from build123d import *

# Parameters (mm, degrees)
SKETCH1_R           = 29.5
BOSS_EXTRUDE1_DEPTH = 1.75
SKETCH2_R           = 27.5
BOSS_EXTRUDE2_DEPTH = 4.45
SKETCH3_R           = 1.25
CUT_EXTRUDE1_DEPTH  = 43.470018837
CIRPATTERN1_COUNT   = 16


with BuildPart() as part:
    # Sketch1 → Boss-Extrude1 (new, symmetric)
    with BuildSketch(Plane(origin=(0, 0, 0), x_dir=(1, 0, 0), z_dir=(0, 1, 0))):
        with Locations(Location((0, 0, 0), (0, 0, 270))):
            Circle(SKETCH1_R)
    extrude(amount=BOSS_EXTRUDE1_DEPTH, both=True)

    # Sketch2 → Boss-Extrude2 (add)
    with BuildSketch(Plane(origin=(0, 1.75, 0), x_dir=(1, 0, 0), z_dir=(0, 1, 0))):
        with Locations(Location((0, 0, 0), (0, 0, 270))):
            Circle(SKETCH2_R)
    extrude(amount=BOSS_EXTRUDE2_DEPTH)

    # Sketch3 → Cut-Extrude1 (cut, through all)
    with BuildSketch(Plane.XZ.offset(1.75)):
        with Locations(Location((0, 23.75, 0), (0, 0, 270))):
            Circle(SKETCH3_R)
    cut_extrude1 = extrude(amount=-CUT_EXTRUDE1_DEPTH, mode=Mode.SUBTRACT)

    # CirPattern1: Cut-Extrude1 ×16 about axis
    cirpattern1_axis = Axis((0, 0, 0), (0, 1, 0))
    for i in range(1, CIRPATTERN1_COUNT):
        add(cut_extrude1.rotate(cirpattern1_axis, i * 360 / CIRPATTERN1_COUNT), mode=Mode.SUBTRACT)


solid = part.part
For this review, take the finished solid that the model builds, in its own axes (mm). A direction names the side the tool comes from. Coordinates: 2 decimals unless noted, no trailing zeros. Write each loop counter-clockwise with the first axis right and the second up, starting at its lowest first coordinate (ties: lowest second). Pieces come first, ordered by that corner, then holes. Notation, with made-up numbers: (50, 80.5) -> (55, 80.5) arc R30 cw to (55, 112.5) -> close; hole circle Ø8 at (30.25, 87.25). An arc over 180 degrees is marked (long way). Write each question's results on one line, items separated by ' | '. Start each with the question number.
1) Consider section C-C (y = -0.5). Give the number of separate pieces and of enclosed holes in the cut face, plus the area to 3 significant figures.
2) Insertion check: pin 1 (1 mm diameter, centred on x = -14, y = 3.5, fed in from -Z); pin 2 (1 mm diameter, centred on x = -16, y = 1, fed in from +Z); pin 3 (1 mm diameter, centred on y = 1.5, z = -1, fed in from +X). Each pin has a flat end and moves straight along its axis. Give the tip position at first contact, or say it passes through.
3) Consider section A-A (x = 0). Write out the cut boundary in (y, z), plus the area to 4 significant figures.
4) Consider section D-D (z = -19.5). Write out the cut boundary in (x, y), plus the area to 3 significant figures.
5) For faces 1 (the face through (15.685, 2.169, -16.216)), 2 (the face through (-24.397, 3.944, 12.69)), list the 3-axis set-ups (+Z, -Z, +X, -X, +Y, -Y) from which the entire face can be reached by the end or side of a thin tool; tool diameter is ignored.
6) The part is to be moulded in two halves that separate along X. For faces 3 (the face through (-20.985, 2.169, -9.893)), 4 (the face through (8.86, 0.02, 28.14)), 5 (the face through (0, -1.75, 0)), say which applies: +X half, -X half, draft (parallel to the pull), parting line (faces both ways), or undercut.
7) Consider section B-B (z = 17). Write out the cut boundary in (x, y).
8) Wall thickness on L1, parallel to Z at x = -8, y = 1.25; L2, parallel to Z at x = 8, y = 5.75; L3, parallel to X at y = 4.75, z = 21: over which ranges is each line inside the solid? List them lowest first. Write a range as [from, to].
Geometry says:
1) separate pieces: 1 | enclosed holes: 16 | area: 2,660 mm^2
2) pin 1: z = -23.96 | pin 2: z = 25.1 | pin 3: x = 29.5
3) outline: (-1.75, -29.5) -> (1.75, -29.5) -> (1.75, -27.5) -> (6.2, -27.5) -> (6.2, -25) -> (-1.75, -25) -> close; (-1.75, -22.5) -> (6.2, -22.5) -> (6.2, 22.5) -> (-1.75, 22.5) -> close; (-1.75, 25) -> (6.2, 25) -> (6.2, 27.5) -> (1.75, 27.5) -> (1.75, 29.5) -> (-1.75, 29.5) -> close | area: 411.5 mm^2
4) outline: (-22.14, -1.75) -> (22.14, -1.75) -> (22.14, 1.75) -> (19.39, 1.75) -> (19.39, 6.2) -> (-19.39, 6.2) -> (-19.39, 1.75) -> (-22.14, 1.75) -> close | area: 328 mm^2
5) face 1: +Y, -Y | face 2: +Y
6) face 3: undercut | face 4: parting line | face 5: draft
7) outline: (-24.11, -1.75) -> (-18.03, -1.75) -> (-18.03, 6.2) -> (-21.62, 6.2) -> (-21.62, 1.75) -> (-24.11, 1.75) -> close; (-15.56, -1.75) -> (15.56, -1.75) -> (15.56, 6.2) -> (-15.56, 6.2) -> close; (18.03, -1.75) -> (24.11, -1.75) -> (24.11, 1.75) -> (21.62, 1.75) -> (21.62, 6.2) -> (18.03, 6.2) -> close
8) L1: [-28.39, -22.56], [-21.33, 21.33], [22.56, 28.39] | L2: [-26.31, -22.56], [-21.33, 21.33], [22.56, 26.31] | L3: [-17.76, -9.91], [-8.27, 8.27], [9.91, 17.76]
